from build123d import *

# Parameters (mm, degrees)
SKETCH1_R           = 6.4
BOSS_EXTRUDE1_DEPTH = 40
SKETCH2_R           = 1.5
CUT_EXTRUDE1_DEPTH  = 1.5
FILLET2_R           = 0.2


with BuildPart() as part:
    # Sketch1 → Boss-Extrude1 (new body)
    with BuildSketch(Plane(origin=(0, 0, 0), x_dir=(1, 0, 0), z_dir=(0, 1, 0))):
        with Locations(Location((0, 0, 0), (0, 0, 270))):
            Circle(SKETCH1_R)
    extrude(amount=BOSS_EXTRUDE1_DEPTH)

    # Sketch2 → Cut-Extrude1 (cut)
    with BuildSketch(Plane(origin=(0, 40, 0), x_dir=(1, 0, 0), z_dir=(0, 1, 0))):
        with Locations(Location((0, 0, 0), (0, 0, 270))):
            Circle(SKETCH2_R)
    cut_extrude1 = extrude(amount=-CUT_EXTRUDE1_DEPTH, mode=Mode.SUBTRACT)

    # Mirror1: Cut-Extrude1 across plane
    add(cut_extrude1.mirror(Plane.ZX.offset(20)), mode=Mode.SUBTRACT)

    # Fillet2
    fillet2_edges = [part.edges().sort_by_distance(p)[0] for p in [
        (0, 0, -1.5),
        (0, 40, -1.5),
    ]]
    fillet(fillet2_edges, radius=FILLET2_R)


solid = part.part
Could you check a few things on this model? Use its own coordinates, in mm. A direction names the side the tool comes from. Give positions to 0.01 mm unless a question says otherwise; leave off trailing zeros. Order: outer loops, then holes, each group sorted by start corner. A loop starts at its lowest first (then second) coordinate and runs counter-clockwise, first axis right, second up.
Item 1: If we section it at C-C, the plane y = 25: Write out the boundary of the cut face in (x, z).
Item 2: For faces 4 (the face through (0.45, 39.16, 1.43)), 5 (the face through (0, 1.5, 0)), 6 (the face through (-1.33, 40, 1.33)), which set-ups out of +Z, -Z, +X, -X, +Y, -Y let a thin tool reach every point of the face, with its end or its side?
Item 3: If we section it at A-A, the plane x = 0: Write out the boundary of the cut face in (y, z).
Item 4: I need wall thicknesses on line 1 (X direction, y = 1.2, z = 0); line 2 (Z direction, x = -0.25, y = 6). Which ranges of each line are inside material? Lowest first, please.
Item 5: If we mould it in two halves opening along X, with no side actions, what happens to faces 1 (the face through (-1.33, 0, 1.33)), 2 (the face through (-3.89, 19.72, -5.08)), 3 (the face through (0.45, 0.84, 1.43))? For each: pulls with the +X half, pulls with the -X half, needs draft (parallel to the pull), parting line crosses it, or undercut.
Item 6: I'm going to push flat-ended pins straight in: pin 1 (4 mm diameter, centred on y = 32.5, z = 4.5, fed in from -X); pin 2 (1 mm diameter, centred on x = -2.5, y = 20.5, fed in from +Z); pin 3 (0.9 mm diameter, centred on x = 0.5, z = 0, fed in from +Y). Where does each tip first touch, or does it pass through?
Item 7: If we section it at D-D, the plane x = -4: Write out the boundary of the cut face in (y, z), plus the area to 3 significant figures.
Item 8: If we section it at B-B, the plane z = 0: Write out the boundary of the cut face in (x, y), plus the area to 3 significant figures.
Values:
1. outline: circle Ø12.8 at (0, 0)
2. face 4: +Y
2. face 5: -Y
2. face 6: +Z, -Z, +X, -X, +Y
3. outline: (0, -6.4) - (40, -6.4) - (40, -1.7) arc R0.2 ccw to (39.8, -1.5) - (38.5, -1.5) - (38.5, 1.5) - (39.8, 1.5) arc R0.2 ccw to (40, 1.7) - (40, 6.4) - (0, 6.4) - (0, 1.7) arc R0.2 ccw to (0.2, 1.5) - (1.5, 1.5) - (1.5, -1.5) - (0.2, -1.5) arc R0.2 ccw to (0, -1.7) - close
4. line 1: x = -6.4 to -1.5, 1.5 to 6.4
4. line 2: z = -6.4 to 6.4
5. face 1: needs draft
5. face 2: parting line crosses it
5. face 3: undercut
6. pin 1: stops at x = -5.89
6. pin 2: stops at z = 6.08
6. pin 3: stops at y = 38.5
7. outline: (0, -5) - (40, -5) - (40, 5) - (0, 5) - close
7. area: 400 mm2
8. outline: (-6.4, 0) - (-1.7, 0) arc R0.2 ccw to (-1.5, 0.2) - (-1.5, 1.5) - (1.5, 1.5) - (1.5, 0.2) arc R0.2 ccw to (1.7, 0) - (6.4, 0) - (6.4, 40) - (1.7, 40) arc R0.2 ccw to (1.5, 39.8) - (1.5, 38.5) - (-1.5, 38.5) - (-1.5, 39.8) arc R0.2 ccw to (-1.7, 40) - (-6.4, 40) - close
8. area: 503 mm2
